The model under review builds one solid part; all positions refer to its coordinate system, in mm. Round coordinates to 2 decimals unless told otherwise and drop trailing zeros. Loops run counter-clockwise (first coordinate to the right, second up) from the corner with the lowest first, then second, coordinate; pieces in that order, holes last. Notation, with made-up numbers: (-20, 19) -> (0, 19) arc R24 cw to (0, 56) -> close; hole circle Ø8 at (58.5, 41.5). An arc over 180 degrees is marked (long way). Write each question's results on one line, items separated by ' | '. Start each with the question number.
Item 1: We need section A-A (y = -1). Give the boundary of the cut face in (x, z), and give its area (3 significant figures).
Item 2: For L1, parallel to Z at x = -51.25, y = -2.3; L2, parallel to Z at x = -56, y = -3.6; L3, parallel to Z at x = -55.25, y = -4.25, list the stretches that pass through material, from the lowest coordinate up. Write a range as from..to.
Item 3: Mouldability with a two-part tool opening along X and no side actions: class faces 1 (the cylindrical face through (-51.853, -2.348, 24.326)), 2 (the flat face through (-48.767, -1.972, 21.155)), 3 (the flat face through (-50.3, 0, 24.6)) as pulls with the +X half, pulls with the -X half, needs draft (parallel to the pull), parting line crosses it, or undercut.
from build123d import *

# Parameters (mm, degrees)
F1_DEPTH = 9.525
F3_R     = 1.6002
F4_DEPTH = 4.7625
F5_R     = 0.762


with BuildPart() as f1:
    # F0 (on Front) → F1 (new body)
    with BuildSketch(Plane.XZ):
        Polygon((-47.0958250334, 35.7042094693), (-47.0958250334, 38.9427094693), (-43.8573250334, 38.9427094693), (-43.8573250334, 41.6986094693), (-49.5457097801, 38.8764154693), (-49.5457097801, 32.5264154693), (-43.8573250334, 29.7042214693), (-43.8573250334, 32.4657094693), (-47.0958250334, 32.4657094693), align=None)
        Polygon((-43.8573250334, 41.6986094693), (-43.8573250334, 38.9427094693), (-40.6188250334, 38.9427094693), (-40.6188250334, 35.7042094693), (-40.6188250334, 32.4657094693), (-43.8573250334, 32.4657094693), (-43.8573250334, 29.7042214693), (-38.1689402867, 32.5264154693), (-38.1689402867, 38.8764154693), align=None)
    extrude(amount=F1_DEPTH)


with BuildPart() as f4:
    # F3 (on Front) → F4 (new body)
    with BuildSketch(Plane.XZ):
        Polygon((-51.5060001731, 32.1294106543), (-57.0622501731, 29.0632774889), (-57.0622501731, 22.7132774889), (-51.5060001731, 19.6390969579), (-45.9497501731, 22.7132774889), (-45.9497501731, 29.0632774889), align=None)
        with Locations((-51.5060001731, 25.8882774889)):
            Circle(F3_R, mode=Mode.SUBTRACT)
    extrude(amount=F4_DEPTH)

    # F5
    f5_edges = [f4.edges().sort_by_distance(p)[0] for p in [
        (-54.284125, -4.7625, 30.596344),
        (-57.06225, -4.7625, 25.888277),
        (-54.284125, -4.7625, 21.176187),
        (-48.727875, -4.7625, 21.176187),
        (-45.94975, -4.7625, 25.888277),
        (-48.727875, -4.7625, 30.596344),
    ]]
    fillet(f5_edges, radius=F5_R)


solid = f4.part
Here are the results:
1) outline: (-57.06, 22.71) -> (-51.51, 19.64) -> (-45.95, 22.71) -> (-45.95, 29.06) -> (-51.51, 32.13) -> (-57.06, 29.06) -> close; hole circle Ø3.2 at (-51.51, 25.89) | area: 96.6 mm2
2) L1: z = 19.78..24.31, 27.47..31.99 | L2: z = 22.13..29.65 | L3: z = 21.76..30.02
3) face 1: undercut | face 2: pulls with the +X half | face 3: needs draft
